Source: three-view drawing plus pictorial views. Frame: mm from the lowest corner of the part. Give positions to 0.01 mm unless a question says otherwise; leave off trailing zeros. Order: outer loops, then holes, each group sorted by start corner. A loop starts at its lowest first (then second) coordinate and runs counter-clockwise, first axis right, second up.
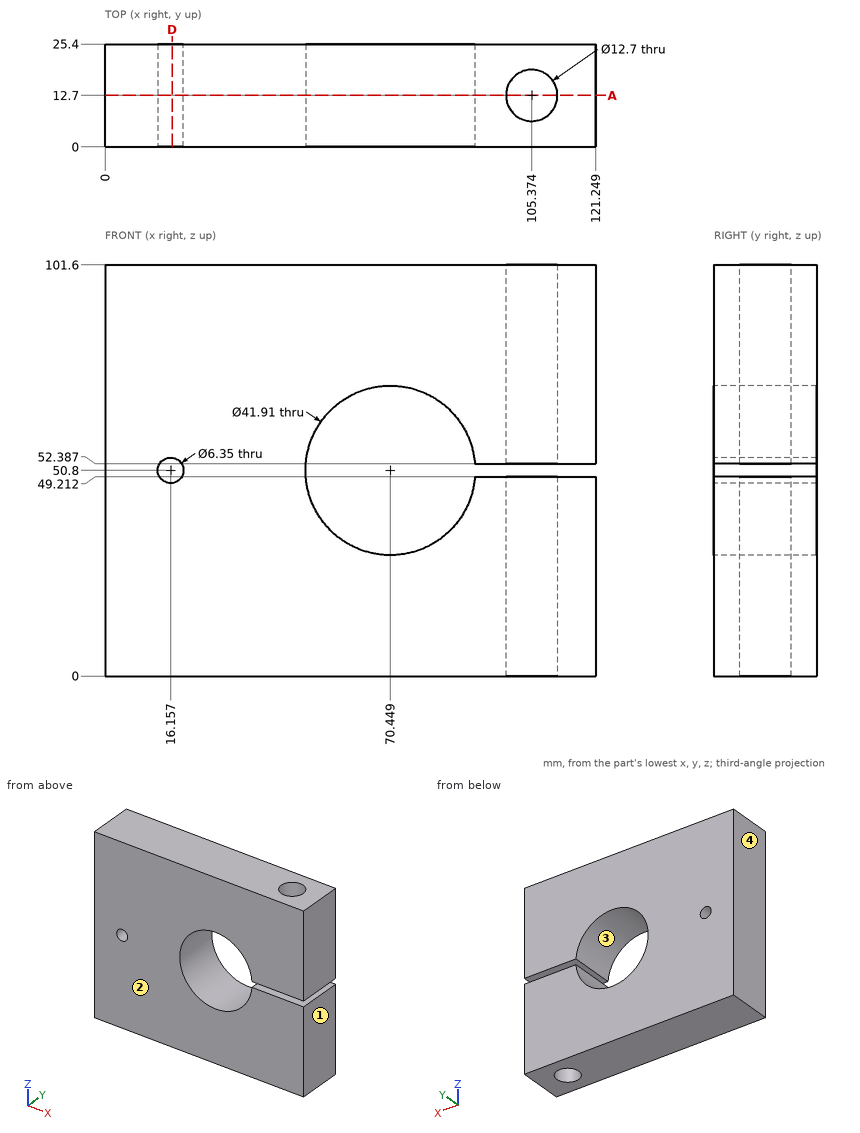
(1) Section A-A, the plane y = 12.7. Count the separate pieces of the cut face and the enclosed holes in it, plus the area to 3 significant figures.
(2) Pin query (flat end, axial travel): pin 1 Ø4 at (x, z) = (16.16, 50.8) entering from -Y. Return the tip coordinate at first contact, or that it passes through.
(3) Section D-D, the plane x = 16.5. Return loops of the section in (y, z), plus the area to 3 significant figures.
(4) Draft query along X for the marked faces 1, 2, 3 and 4. Return one class per face: +X half, -X half, draft (parallel to the pull), parting line (faces both ways), or undercut.
(5) Line query: line 1 along Z through (x, y) = (115, 18.5); line 2 along Z through (x, y) = (62, 14.25) (1 decimal); line 3 along X through (y, z) = (6.5, 49.5) (1 decimal). Output: solid intervals per line, ascending.
Checks:
1. separate pieces: 3
1. enclosed holes: 1
1. area: 9,560 mm2
2. pin 1: passes through
3. outline: (0, 0) - (25.4, 0) - (25.4, 47.64) - (0, 47.64) - close; (0, 53.96) - (25.4, 53.96) - (25.4, 101.6) - (0, 101.6) - close
3. area: 2,420 mm2
4. face 1: +X half
4. face 2: draft
4. face 3: undercut
4. face 4: -X half
5. line 1: z = 0 to 49.21, 52.39 to 101.6
5. line 2: z = 0 to 31.6, 70 to 101.6
5. line 3: x = 0 to 13.3, 19.1 to 49.5
